Read the model definition and answer for the solid it produces. Units are mm, in the model's axes. Face numbers are marked on the shaded views. Coordinates: 2 decimals unless noted, no trailing zeros. Loops run counter-clockwise (first coordinate to the right, second up) from the corner with the lowest first, then second, coordinate; pieces in that order, holes last. Notation, with made-up numbers: (38.25, 19) - (45.25, 19) arc R8 ccw to (45.25, 25) - close; hole circle Ø9 at (-2, 14.25). An arc over 180 degrees is marked (long way). Use one line per item in the form item = value.
Autodesk Fusion 360 part; units mm, degrees
sketch "Sketch1" plane through (0, 0, 0) normal (0, 0, 1) x (1, 0, 0)
  line L0 (30, -10) -> (-30, -10)
  line L1 (-30, -10) -> (-30, 10)
  line L2 (-30, 10) -> (30, 10)
  line L3 (30, 10) -> (30, -10)
  line L4 (30, -10) -> (-30, 10) construction
  line L5 (-30, -10) -> (30, 10) construction
  dimension "d1" = 60
  dimension "d2" = 20
extrude "Extrude1" add sketch "Sketch1" along normal blind 1
sketch "Sketch2" plane through (0, 0, 0) normal (1, 0, 0) x (0, 1, 0)
  line L0 (5.5, 1) -> (2.813, 3.687)
  line L1 (5.5, 1) -> (9.3, 1) construction
  line L2 (2.813, 3.687) -> (5.813, 3.687)
  line L3 (5.813, 3.687) -> (8.5, 1)
  line L4 (-5.5, 1) -> (-2.813, 3.687)
  line L5 (-5.813, 3.687) -> (-8.5, 1)
  line L6 (-2.813, 3.687) -> (-5.813, 3.687)
  line L7 (-8.5, 1) -> (-5.5, 1)
  line L8 (5.5, 1) -> (8.5, 1)
extrude "Extrude2" add sketch "Sketch2" along normal mid plane 25
fillet "Fillet1" radius 3 2 edges at (0, -8.5, 1) (0, 8.5, 1)
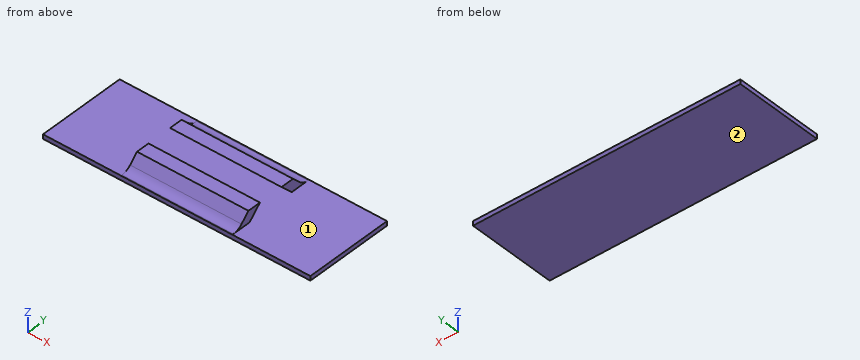
Item 1: The part is cut by section D-D on y = -7. Give the vertices of the cut face in (x, z), plus the area to 3 significant figures.
Results below:
outline = (-30, 0) - (30, 0) - (30, 1) - (12.5, 1) - (12.5, 2.5) - (-12.5, 2.5) - (-12.5, 1) - (-30, 1) - close
area = 97.5 mm²
Item 2: Each of these flat-tipped pins is pushed along its axis until it touches: P1, Ø1.3, axis at y = -5.5, z = 2, coming from the +X side; P2, Ø1, axis at x = 16, z = 2.5, coming from the +Y side; P3, Ø2, axis at y = -5, z = 2.5, coming from the -X side. Where does it stop, or does it pass through?
Results below:
P1 = 12.5
P2 = through
P3 = -12.5
Item 3: Find the intervals of material crossed by L1, parallel to Z at x = -26, y = 2.75; L2, parallel to Y at x = -2.5, z = 2.05; L3, parallel to Y at x = 7.5, z = 2.8, in increasing order.
Results below:
L1 = 0 to 1
L2 = -7.45 to -4.45, 4.45 to 7.45
L3 = -6.7 to -3.7, 3.7 to 6.7
Item 4: For a pull along Y with two mould halves and no side action, classify the marked faces 1 and 2 as +Y half, -Y half, draft (parallel to the pull), parting line (faces both ways), or undercut.
Results below:
face_1 = undercut
face_2 = draft
Item 5: The part is cut by section B-B on z = 2.8. Give the vertices of the cut face in (x, y), plus the area to 3 significant figures.
Results below:
outline = (-12.5, -6.7) - (12.5, -6.7) - (12.5, -3.7) - (-12.5, -3.7) - close; (-12.5, 3.7) - (12.5, 3.7) - (12.5, 6.7) - (-12.5, 6.7) - close
area = 150 mm²
Item 6: The part is cut by section A-A on y = 4. Give the vertices of the cut face in (x, z), plus the area to 3 significant figures.
Results below:
outline = (-30, 0) - (30, 0) - (30, 1) - (-30, 1) - close; (-12.5, 2.5) - (12.5, 2.5) - (12.5, 3.69) - (-12.5, 3.69) - close
area = 89.7 mm²
Item 7: The part is cut by section C-C on x = 7.5. Give the vertices of the cut face in (y, z).
Results below:
outline = (-10, 0) - (10, 0) - (10, 1) - (9.74, 1) arc R3 cw to (7.62, 1.88) - (5.81, 3.69) - (2.81, 3.69) - (5.5, 1) - (-5.5, 1) - (-2.81, 3.69) - (-5.81, 3.69) - (-7.62, 1.88) arc R3 cw to (-9.74, 1) - (-10, 1) - close
